Part model, mm, in its own coordinate system. Face numbers are marked on the shaded views. A direction names the side the tool comes from. Coordinates: 2 decimals unless noted, no trailing zeros. Loops run counter-clockwise (first coordinate to the right, second up) from the corner with the lowest first, then second, coordinate; pieces in that order, holes last. Notation, with made-up numbers: (42.25, 64.5) - (53.25, 64.5) arc R14 cw to (53.25, 87.5) - close; hole circle Ø3 at (-6.5, -37). An arc over 180 degrees is marked (long way). Use a Markdown table: item, result. Add a question column.
1. 3-axis set-ups, long thin cutter, end or side, ignore diameter. For the marked faces 5 and 6: which of +Z, -Z, +X, -X, +Y, -Y reach the whole face in a straight line?
2. Pull direction X, two halves, no side cores. Call the marked faces 1, 2, 3 and 4: pulls with the +X half, pulls with the -X half, needs draft (parallel to the pull), parting line crosses it, or undercut.
3. Drop flat-ended pins along their axis: pin 1 (2.5 mm diameter, centred on x = 106.5, z = -15.5, fed in from +Y); pin 2 (2.5 mm diameter, centred on x = 107.5, z = 10.5, fed in from -Y); pin 3 (6 mm diameter, centred on y = -25, z = 47.43, fed in from -X); pin 4 (8 mm diameter, centred on x = 26, y = -50, fed in from +Z). Give the stop position or say it passes through.
4. Band-saw the part on A-A, the plane z = 3.5. Give the cut face in (x, y).
5. Band-saw the part on D-D, the plane y = -4.5. Give the cut face in (x, z), plus the area to 3 significant figures.
6. Wall check: probe 1 along X at (y, z) = (-45, -13.5); probe 2 along Z at (x, y) = (-88, -48). Give the ranges that are in metal, low to high. Write a range as [from, to].
7. Band-saw the part on C-C, the plane y = -54. Give the cut face in (x, z).
8. Band-saw the part on B-B, the plane x = -56. Give the cut face in (y, z), plus the area to 3 significant figures.
from build123d import *

# Parameters (mm, degrees)
F1_DEPTH = 50
F2_R     = 24.99999
F3_R     = 5
F4_DEPTH = 230.001
F6_DEPTH = 5


# Not quite as in the source:
# - a fillet or chamfer is up to 0.001 mm smaller than in the source, because OpenCascade refuses the exact size


with BuildPart() as f1:
    # F0 (on Front) → F1 (new body)
    with BuildSketch(Plane.XZ):
        Polygon((-119.9185385572, 72.4322550792), (-119.9185385572, -82.5677449208), (110.0814614428, -82.5677449208), (110.0814614428, 72.4322550792), (105.0814614428, 72.4322550792), (105.0814614428, -77.5677449208), (-114.9185385572, -77.5677449208), (-114.9185385572, 72.4322550792), align=None)
    extrude(amount=F1_DEPTH)

    # F2 (radius 25 in the source; OpenCascade refuses exactly that, so slightly less here)
    f2_edges = [f1.edges().sort_by_distance(p)[0] for p in [
        (-117.418539, -50, 72.432255),
        (-117.418539, 0, 72.432255),
        (107.581461, -50, 72.432255),
        (107.581461, 0, 72.432255),
    ]]
    fillet(f2_edges, radius=F2_R)

    # F3 (on face) → F4 (cut, through all)
    with BuildSketch(Plane(origin=(-119.9185385572, 0, 0), x_dir=(0, -1, 0), z_dir=(-1, 0, 0))):
        with Locations((25, 47.4322550792)):
            Circle(F3_R)
    extrude(amount=-F4_DEPTH, mode=Mode.SUBTRACT)

    # F5 (on face) → F6 (join)
    with BuildSketch(Plane(origin=(0, 0, -82.5677449208), x_dir=(1, 0, 0), z_dir=(0, 0, -1))):
        with BuildLine():
            Line((80.0814614428, 105), (-89.9185385572, 105))
            ThreePointArc((-89.9185385572, 105), (-111.1317419928, 96.2132034356), (-119.9185385572, 75))
            Line((-119.9185385572, 75), (-119.9185385572, -25))
            ThreePointArc((-119.9185385572, -25), (-111.1317419928, -46.2132034356), (-89.9185385572, -55))
            Line((-89.9185385572, -55), (80.0814614428, -55))
            ThreePointArc((80.0814614428, -55), (101.2946648784, -46.2132034356), (110.0814614428, -25))
            Line((110.0814614428, -25), (110.0814614428, 75))
            ThreePointArc((110.0814614428, 75), (101.2946648784, 96.2132034356), (80.0814614428, 105))
        make_face()
    extrude(amount=-F6_DEPTH)


solid = f1.part
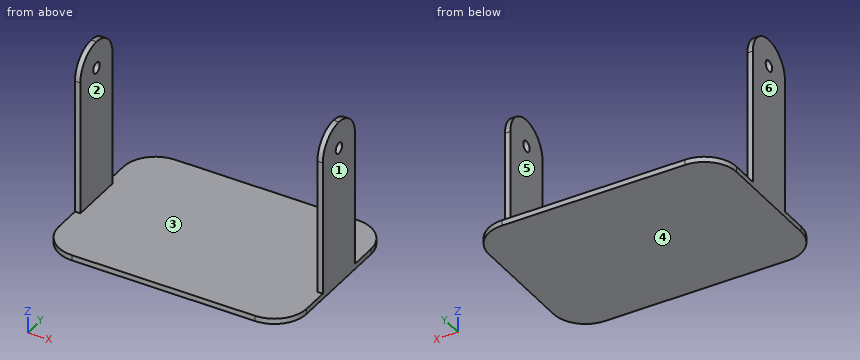
Geometry check:
| question | item | result |
|---|---|---|
| 1 | face 5 | +Z, +Y, -Y |
| 1 | face 6 | +Z, -Z, -X, +Y, -Y |
| 2 | face 1 | pulls with the +X half |
| 2 | face 2 | undercut |
| 2 | face 3 | undercut |
| 2 | face 4 | needs draft |
| 3 | pin 1 | stops at y = 0 |
| 3 | pin 2 | stops at y = -50 |
| 3 | pin 3 | passes through |
| 3 | pin 4 | stops at z = -77.57 |
| 4 | outline | (-119.92, -50) - (-114.92, -50) - (-114.92, 0) - (-119.92, 0) - close; (105.08, -50) - (110.08, -50) - (110.08, 0) - (105.08, 0) - close |
| 5 | outline | (-119.92, -82.57) - (110.08, -82.57) - (110.08, 61.74) - (105.08, 61.74) - (105.08, -77.57) - (-114.92, -77.57) - (-114.92, 61.74) - (-119.92, 61.74) - close |
| 5 | area | 2,540 mm^2 |
| 6 | probe 1 | x = [-119.92, -114.92], [105.08, 110.08] |
| 6 | probe 2 | z = [-82.57, -77.57] |
| 7 | outline | (-119.92, -82.57) - (110.08, -82.57) - (110.08, -77.57) - (-119.92, -77.57) - close |
| 8 | outline | (-105, -82.57) - (55, -82.57) - (55, -77.57) - (-105, -77.57) - close |
| 8 | area | 800 mm^2 |
